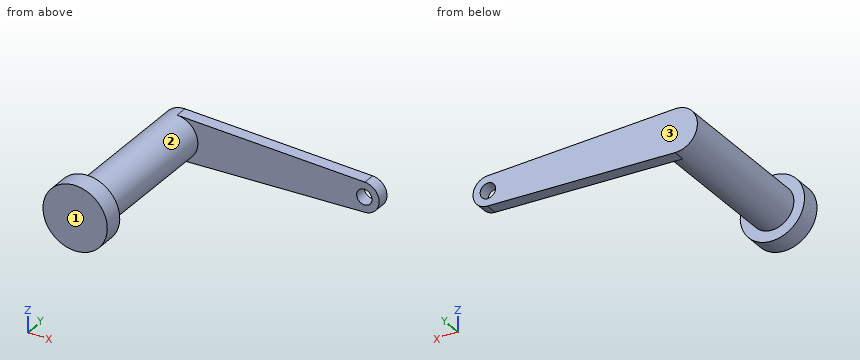
```python
from build123d import *

# Parameters (mm, degrees)
SKETCH_2_R          = 1.5
CUT_EXTRUDE_5_DEPTH = 10
SKETCH_3_R          = 2.5
EXTRUDE_1_DEPTH     = 20
SKETCH_4_R          = 1.85
EXTRUDE_2_DEPTH     = 5
SKETCH_3_2_R        = 2.5
EXTRUDE_3_DEPTH     = 5.891507394
SKETCH_5_R          = 4.35
EXTRUDE_4_DEPTH     = 25
SKETCH_6_R          = 6.5
EXTRUDE_5_DEPTH     = 4
SKETCH_7_OUTSIDE_W  = 65.264
SKETCH_7_OUTSIDE_H  = 65.264
CUT_EXTRUDE_6_DEPTH = 5
SKETCH_8_R          = 1.55
EXTRUDE_6_DEPTH     = 2.5


with BuildPart() as part:
    # Sketch 1 → Revolve 1 (revolve)
    with BuildSketch(Plane.XY, mode=Mode.PRIVATE) as revolve_1_sk:
        Polygon((3.461552813, 5.891507394), (1.4, 5.891507394), (1.4, 3.5), (2.5, 3.5), (2.5, 0), (4.35, 0), (4.35, 3.391507394), (24, 3.391507394), (24, 5.891507394), align=None)
    revolve(revolve_1_sk.sketch.rotate(Axis((0, 0, 0), (0, 1, 0)), 90), axis=Axis((0, 0, 0), (0, 1, 0)))

    # Sketch 2 → Cut-Extrude 5 (cut)
    with BuildSketch(Plane(origin=(0, 5.891507394, 0), x_dir=(1, 0, 0), z_dir=(0, 1, 0))):
        with Locations(Location((-16, 0, 0), (0, 0, 270))):
            Circle(SKETCH_2_R)
        with Locations(Location((0, -16, 0), (0, 0, 270))):
            Circle(SKETCH_2_R)
        with Locations(Location((16, 0, 0), (0, 0, 270))):
            Circle(SKETCH_2_R)
        with Locations(Location((0, 16, 0), (0, 0, 270))):
            Circle(SKETCH_2_R)
    extrude(amount=-CUT_EXTRUDE_5_DEPTH, mode=Mode.SUBTRACT)



with BuildPart() as body_2:
    # Sketch 3 → Extrude 1 (new body)
    with BuildSketch(Plane.XZ):
        with Locations(Location((0, 0, 0), (0, 0, 270))):
            Circle(SKETCH_3_R)
    extrude(amount=EXTRUDE_1_DEPTH)

    # Sketch 4 → Extrude 2 (add)
    with BuildSketch(Plane.XZ.offset(20)):
        with Locations(Location((0, 0, 0), (0, 0, 270))):
            Circle(SKETCH_4_R)
    extrude(amount=EXTRUDE_2_DEPTH)


with BuildPart() as part_1:
    add(part.part)

    add(body_2.part)  # Extrude 3 merges body 2
    # Sketch 3_2 → Extrude 3 (add)
    with BuildSketch(Plane.XZ):
        with Locations(Location((0, 0, 0), (0, 0, 270))):
            Circle(SKETCH_3_2_R)
    extrude(amount=-EXTRUDE_3_DEPTH)

    # Sketch 5 → Extrude 4 (add, through all)
    with BuildSketch(Plane.XZ):
        with Locations(Location((0, 0, 0), (0, 0, 270))):
            Circle(SKETCH_5_R)
    extrude(amount=EXTRUDE_4_DEPTH)

    # Sketch 6 → Extrude 5 (add)
    with BuildSketch(Plane.XZ.offset(25)):
        with Locations(Location((0, 0, 0), (0, 0, 270))):
            Circle(SKETCH_6_R)
    extrude(amount=EXTRUDE_5_DEPTH)

    # Sketch 7 outside → Cut-Extrude 6 (cut)
    with BuildSketch(Plane(origin=(0, 5.891507394, 0), x_dir=(1, 0, 0), z_dir=(0, 1, 0))):
        Rectangle(SKETCH_7_OUTSIDE_W, SKETCH_7_OUTSIDE_H)
        with BuildLine():
            Line((0.36703125, 4.334488212), (16.253125, 2.989302215))
            ThreePointArc((16.253125, 2.989302215), (19, 0), (16.253125, -2.989302215))
            Line((16.253125, -2.989302215), (0.36703125, -4.334488212))
            ThreePointArc((0.36703125, -4.334488212), (-4.35, 0), (0.36703125, 4.334488212))
        make_face(mode=Mode.SUBTRACT)
    extrude(amount=-CUT_EXTRUDE_6_DEPTH, mode=Mode.SUBTRACT)

    # Sketch 8 → Extrude 6 (add)
    with BuildSketch(Plane(origin=(0, 5.891507394, 0), x_dir=(1, 0, 0), z_dir=(0, 1, 0))):
        with BuildLine():
            Line((0.154539474, 4.347254024), (38.106578947, 2.998106224))
            ThreePointArc((38.106578947, 2.998106224), (41, 0), (38.106578947, -2.998106224))
            Line((38.106578947, -2.998106224), (0.154539474, -4.347254024))
            ThreePointArc((0.154539474, -4.347254024), (-4.35, 0), (0.154539474, 4.347254024))
        make_face()
        with Locations(Location((38, 0, 0), (0, 0, 270))):
            Circle(SKETCH_8_R, mode=Mode.SUBTRACT)
    extrude(amount=-EXTRUDE_6_DEPTH)


solid = part_1.part
```
Geometry check sheet. Reference: the model listing, model coordinates, mm. Face numbers are marked on the shaded views. Give positions to 0.01 mm unless a question says otherwise; leave off trailing zeros. Write each loop counter-clockwise with the first axis right and the second up, starting at its lowest first coordinate (ties: lowest second). Pieces come first, ordered by that corner, then holes. Notation, with made-up numbers: (29.25, 47) - (78.25, 47) arc R24 ccw to (78.25, 73) - close; hole circle Ø8 at (21.5, 58). An arc over 180 degrees is marked (long way). Use a Markdown table: item, result.
Q1. Thickness scan on L1, parallel to X at y = 5.2, z = 0; L2, parallel to Y at x = 5, z = 1.25; L3, parallel to Y at x = 23, z = -3. Record the ranges inside material, lowest first. Write a range as [from, to].
Computed:
| item | result |
|---|---|
| L1 | x = [-4.35, 36.45], [39.55, 41] |
| L2 | y = [-29, -25], [3.39, 5.89] |
| L3 | y = [3.39, 5.89] |
Q2. Section check C-C, the plane x = 2. Enter the section's corners in (y, z).
Computed:
| item | result |
|---|---|
| outline | (-29, -6.18) - (-25, -6.18) - (-25, -3.86) - (3.39, -3.86) - (3.39, -4.28) - (5.89, -4.28) - (5.89, 4.28) - (3.39, 4.28) - (3.39, 3.86) - (-25, 3.86) - (-25, 6.18) - (-29, 6.18) - close |
Q3. Section check B-B, the plane y = 4. Enter the section's corners in (x, z).
Computed:
| item | result |
|---|---|
| outline | (0.15, -4.35) - (38.11, -3) arc R3 ccw to (38.11, 3) - (0.15, 4.35) arc R4.35 ccw (long way) to start; hole circle Ø3.1 at (38, 0) |
Q4. Draft check along Y on the marked faces 1, 2 and 3. Enter one of: pulls with the +Y half, pulls with the -Y half, needs draft (parallel to the pull), parting line crosses it, or undercut.
Computed:
| item | result |
|---|---|
| face 1 | pulls with the -Y half |
| face 2 | undercut |
| face 3 | pulls with the +Y half |
Q5. Go/stop test with flat-tipped pins: P1, Ø6, axis at x = 17, z = -4, coming from the -Y side; P2, Ø10, axis at x = 4.5, y = -18.5, coming from the +Z side; P3, Ø3, axis at x = 5.5, y = -16.5, coming from the -Z side. Record where each tip stops, or that it passes through.
Computed:
| item | result |
|---|---|
| P1 | stops at y = 3.39 |
| P2 | stops at z = 4.35 |
| P3 | stops at z = -1.71 |
Q6. Section check A-A, the plane z = 0. Enter the section's corners in (x, y), then the cut area to 3 significant figures.
Computed:
| item | result |
|---|---|
| outline | (-6.5, -29) - (6.5, -29) - (6.5, -25) - (4.35, -25) - (4.35, 3.39) - (36.45, 3.39) - (36.45, 5.89) - (-4.35, 5.89) - (-4.35, -25) - (-6.5, -25) - close; (39.55, 3.39) - (41, 3.39) - (41, 5.89) - (39.55, 5.89) - close |
| area | 405 mm² |
Q7. Section check D-D, the plane y = -18.5. Enter the section's corners in (x, z), then the cut area to 3 significant figures.
Computed:
| item | result |
|---|---|
| outline | circle Ø8.7 at (0, 0) |
| area | 59.4 mm² |
